The figure shows three views and two pictorial views of one solid part (mm, origin at its lowest corner). Answer the questions. Round coordinates to 2 decimals unless told otherwise and drop trailing zeros. Order: outer loops, then holes, each group sorted by start corner. A loop starts at its lowest first (then second) coordinate and runs counter-clockwise, first axis right, second up. Notation, with made-up numbers: (6.25, 64.25) -> (49.25, 64.25) arc R6 cw to (49.25, 69.25) -> close; hole circle Ø8 at (-17.75, 6). An arc over 180 degrees is marked (long way). One line per item, written item: value. Start each with the question number.
1. Section A-A (x = 25) is taken. Give the vertices of the cut face in (y, z), then the cut area to 3 significant figures.
2. Consider line 1 (X direction, y = 12, z = 1.35); line 2 (Y direction, x = 25, z = 1.95); line 3 (X direction, y = 38.5, z = 0.95). Determine where each line is inside the solid, lowest interval first.
3. Section D-D (x = 42) is taken. Give the vertices of the cut face in (y, z).
4. Section C-C (z = 1.5) is taken. Give the vertices of the cut face in (x, y) (3 decimals).
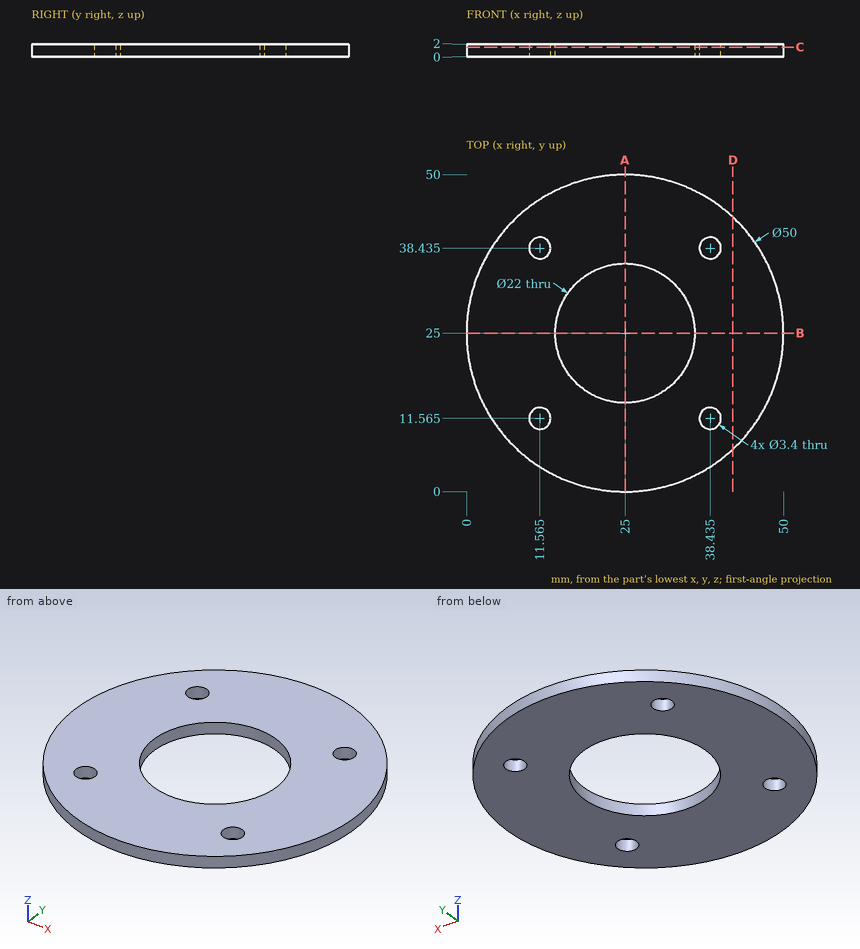
Answer:
1. outline: (0, 0) -> (14, 0) -> (14, 2) -> (0, 2) -> close; (36, 0) -> (50, 0) -> (50, 2) -> (36, 2) -> close
1. area: 56.0 mm^2
2. line 1: 3.65 to 9.92, 13.21 to 36.79, 40.08 to 46.35
2. line 2: 0 to 14, 36 to 50
2. line 3: 3.96 to 9.87, 13.26 to 36.74, 40.13 to 46.04
3. outline: (6.67, 0) -> (43.33, 0) -> (43.33, 2) -> (6.67, 2) -> close
4. outline: circle Ø50 at (25, 25); hole circle Ø3.4 at (11.565, 11.565); hole circle Ø3.4 at (11.565, 38.435); hole circle Ø22 at (25, 25); hole circle Ø3.4 at (38.435, 11.565); hole circle Ø3.4 at (38.435, 38.435)
